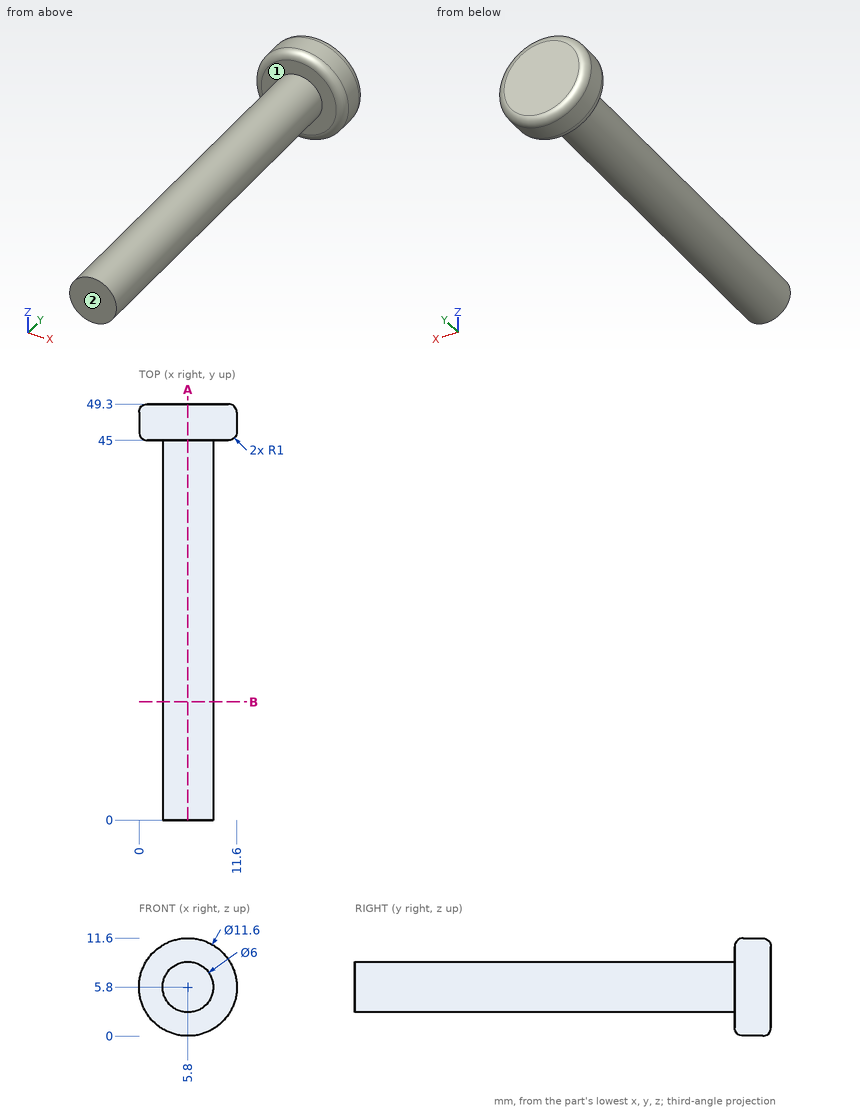
Can you work these out from the drawing? Everything is in mm from the part's minimum corner. A direction names the side the tool comes from. Coordinates: 2 decimals unless noted, no trailing zeros. Write each loop counter-clockwise with the first axis right and the second up, starting at its lowest first coordinate (ties: lowest second). Pieces come first, ordered by that corner, then holes. Notation, with made-up numbers: (-4.5, 87.5) -> (22.5, 87.5) arc R25 cw to (22.5, 120.5) -> close; hole circle Ø2 at (-27, 83). An arc over 180 degrees is marked (long way). Write each question's results on one line, items separated by ' | '. Start each with the question number.
Q1. Imagine slicing it at B-B (y = 14). Write out the boundary of the cut face in (x, z), then the cut area to 3 significant figures.
Q2. If I drill on probe 1 along Y at (x, z) = (9.25, 7); probe 2 along Z at (x, y) = (5.75, 44.5); probe 3 along X at (y, z) = (20, 4.25), over which ranges is the centre line in solid material (lowest first)?
Q3. I'm going to push flat-ended pins straight in: pin 1 (5 mm diameter, centred on x = 2.5, y = 30.5, fed in from -Z); pin 2 (4 mm diameter, centred on y = 13.5, z = 7, fed in from -X); pin 3 (3 mm diameter, centred on x = 6, z = 6.5, fed in from -Y); pin 4 (4 mm diameter, centred on y = 43.5, z = 3, fed in from -X). Where does each tip first touch, or does it pass through?
Q4. On a 3-axis mill with a long thin cutter (end or side, diameter ignored), from which of +Z, -Z, +X, -X, +Y, -Y can I reach the whole of each face in a straight line? I mean the marked faces 1 and 2. Say none if no direction works.
Q5. Imagine slicing it at A-A (x = 5.8). Write out the boundary of the cut face in (y, z), then the cut area to 3 significant figures.
Taken from the geometry:
1) outline: circle Ø6 at (5.8, 5.8) | area: 28.3 mm^2
2) probe 1: y = 45 to 49.3 | probe 2: z = 2.8 to 8.8 | probe 3: x = 3.23 to 8.37
3) pin 1: stops at z = 2.91 | pin 2: stops at x = 2.8 | pin 3: stops at y = 0 | pin 4: stops at x = 0.63
4) face 1: -Y | face 2: +Z, -Z, +X, -X, -Y
5) outline: (0, 2.8) -> (45, 2.8) -> (45, 1) arc R1 ccw to (46, 0) -> (48.3, 0) arc R1 ccw to (49.3, 1) -> (49.3, 10.6) arc R1 ccw to (48.3, 11.6) -> (46, 11.6) arc R1 ccw to (45, 10.6) -> (45, 8.8) -> (0, 8.8) -> close | area: 319 mm^2
